The drawing under review shows one solid part. Ordinate dimensions are in mm from its lowest x, y, z. A direction names the side the tool comes from. Coordinates: 2 decimals unless noted, no trailing zeros. Loops run counter-clockwise (first coordinate to the right, second up) from the corner with the lowest first, then second, coordinate; pieces in that order, holes last. Notation, with made-up numbers: (-3, -40) -> (30, -40) arc R15 ccw to (30, -23) -> close; hole circle Ø1 at (-21, 21). An arc over 180 degrees is marked (long way). Use a Markdown table: item, result.
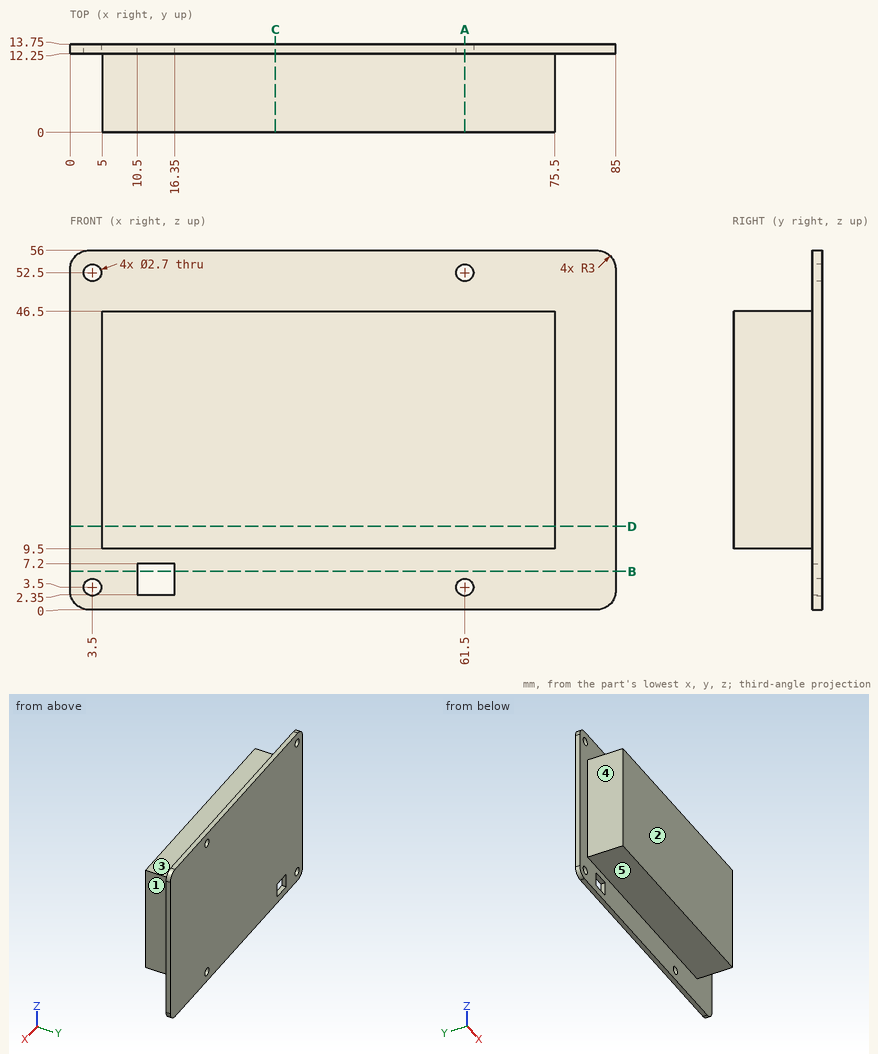
(1) Take a section at C-C on x = 32. Write out the cut boundary in (y, z), plus the area to 3 significant figures.
Found:
| item | result |
|---|---|
| outline | (0, 9.5) -> (12.25, 9.5) -> (12.25, 0) -> (13.75, 0) -> (13.75, 56) -> (12.25, 56) -> (12.25, 46.5) -> (0, 46.5) -> close |
| area | 537 mm^2 |
(2) For pin 1 Ø3 at (x, z) = (61.5, 3.5) entering from -Y; pin 2 Ø1.5 at (x, y) = (71.5, 10.5) entering from +Z; pin 3 Ø3.5 at (y, z) = (6, 26.5) entering from +X, all flat-tipped, find the tip position at first contact; note any pin that passes through.
Found:
| item | result |
|---|---|
| pin 1 | stops at y = 12.25 |
| pin 2 | stops at z = 46.5 |
| pin 3 | stops at x = 75.5 |
(3) Take a section at A-A on x = 61.5. Write out the cut boundary in (y, z).
Found:
| item | result |
|---|---|
| outline | (0, 9.5) -> (12.25, 9.5) -> (12.25, 4.85) -> (13.75, 4.85) -> (13.75, 51.15) -> (12.25, 51.15) -> (12.25, 46.5) -> (0, 46.5) -> close; (12.25, 0) -> (13.75, 0) -> (13.75, 2.15) -> (12.25, 2.15) -> close; (12.25, 53.85) -> (13.75, 53.85) -> (13.75, 56) -> (12.25, 56) -> close |
(4) Take a section at D-D on z = 13. Write out the cut boundary in (x, y), plus the area to 3 significant figures.
Found:
| item | result |
|---|---|
| outline | (0, 12.25) -> (5, 12.25) -> (5, 0) -> (75.5, 0) -> (75.5, 12.25) -> (85, 12.25) -> (85, 13.75) -> (0, 13.75) -> close |
| area | 991 mm^2 |
(5) For line 1 along Z through (x, y) = (3.5, 13); line 2 along Z through (x, y) = (25, 9); line 3 along X through (y, z) = (9.75, 44.5), list the stretches that pass through material, from the lowest coordinate up.
Found:
| item | result |
|---|---|
| line 1 | z = 0 to 2.15, 4.85 to 51.15, 53.85 to 56 |
| line 2 | z = 9.5 to 46.5 |
| line 3 | x = 5 to 75.5 |
(6) Take a section at B-B on z = 6. Write out the cut boundary in (x, y).
Found:
| item | result |
|---|---|
| outline | (0, 12.25) -> (10.5, 12.25) -> (10.5, 13.75) -> (0, 13.75) -> close; (16.35, 12.25) -> (85, 12.25) -> (85, 13.75) -> (16.35, 13.75) -> close |
(7) For the marked faces 1, 2, 3, 4 and 5, list the 3-axis set-ups (+Z, -Z, +X, -X, +Y, -Y) from which the entire face can be reached by the end or side of a thin tool; tool diameter is ignored.
Found:
| item | result |
|---|---|
| face 1 | +Z, -Z, +X, -Y |
| face 2 | +Z, -Z, +X, -X, -Y |
| face 3 | +Z, +X, -X, -Y |
| face 4 | +Z, -Z, -X, -Y |
| face 5 | -Z, +X, -X, -Y |
